```python
from build123d import *

# Parameters (mm, degrees)
SKETCH1_R                = 2.5
BOSS_EXTRUDE3_DEPTH      = 6.5
BOSS_EXTRUDE3_2_DEPTH    = 6.5
BOSS_EXTRUDE7_START      = -6.5
BOSS_EXTRUDE7_DEPTH      = 1.5
BOSS_EXTRUDE8_DEPTH      = 8.5
BOSS_EXTRUDE8_DEPTH_BACK = 8.5
SKETCH2_R                = 2.5
SKETCH3_R                = 1.5
CUT_EXTRUDE1_DEPTH       = 0.5
CUT_EXTRUDE2_START       = -0.5
SKETCH4_R                = 1.5
CUT_EXTRUDE2_DEPTH       = 0.5


with BuildPart() as part:
    # Sketch1 → Boss-Extrude3 (new, symmetric)
    with BuildSketch(Plane.XY):
        with Locations(Location((6.35, 0, 0), (0, 0, 180))):
            Circle(SKETCH1_R)
    extrude(amount=BOSS_EXTRUDE3_DEPTH, both=True)



with BuildPart() as body_2:
    # Sketch1 → Boss-Extrude3 2 (new, symmetric)
    with BuildSketch(Plane.XY):
        with Locations(Location((-6.35, 0, 0), (0, 0, 180))):
            Circle(SKETCH1_R)
    extrude(amount=BOSS_EXTRUDE3_2_DEPTH, both=True)


with BuildPart() as part_1:
    add(part.part)

    add(body_2.part)  # Boss-Extrude7 merges body 2
    # Sketch1<5> → Boss-Extrude7 (add)
    with BuildSketch(Plane.XY.offset(BOSS_EXTRUDE7_START)):
        with BuildLine():
            ThreePointArc((-3.267678659, 4.854049356), (-12.1, 0), (-3.267678659, -4.854049356))
            ThreePointArc((-3.267678659, -4.854049356), (0, -3.904220161), (3.267678659, -4.854049356))
            ThreePointArc((3.267678659, -4.854049356), (12.1, 0), (3.267678659, 4.854049356))
            ThreePointArc((3.267678659, 4.854049356), (0, 3.904220161), (-3.267678659, 4.854049356))
        make_face()
    boss_extrude7 = extrude(amount=-BOSS_EXTRUDE7_DEPTH)

    # Mirror1: Boss-Extrude7 across plane
    add(boss_extrude7.mirror(Plane.XY))

    # Sketch2 → Boss-Extrude8 (add, two sides: drawn at the far end of the back side and taken through both)
    with BuildSketch(Plane.XY.offset(-BOSS_EXTRUDE8_DEPTH_BACK)):
        with Locations(Location((-6.35, 0, 0), (0, 0, 180))):
            Circle(SKETCH2_R)
        with Locations(Location((6.35, 0, 0), (0, 0, 180))):
            Circle(SKETCH2_R)
    extrude(amount=BOSS_EXTRUDE8_DEPTH + BOSS_EXTRUDE8_DEPTH_BACK)

    # Sketch3 → Cut-Extrude1 (cut)
    with BuildSketch(Plane.XY.offset(8.5)):
        with Locations((-6.35, 0)):
            Circle(SKETCH3_R)
        with Locations((6.35, 0)):
            Circle(SKETCH3_R)
    extrude(amount=-CUT_EXTRUDE1_DEPTH, mode=Mode.SUBTRACT)

    # Sketch4 → Cut-Extrude2 (cut)
    with BuildSketch(Plane(origin=(0, 0, -8.5), x_dir=(-1, 0, 0), z_dir=(0, 0, -1)).offset(CUT_EXTRUDE2_START)):
        with Locations(Location((6.35, 0, 0), (0, 0, 180))):
            Circle(SKETCH4_R)
        with Locations(Location((-6.35, 0, 0), (0, 0, 180))):
            Circle(SKETCH4_R)
    extrude(amount=CUT_EXTRUDE2_DEPTH, mode=Mode.SUBTRACT)


solid = part_1.part
```
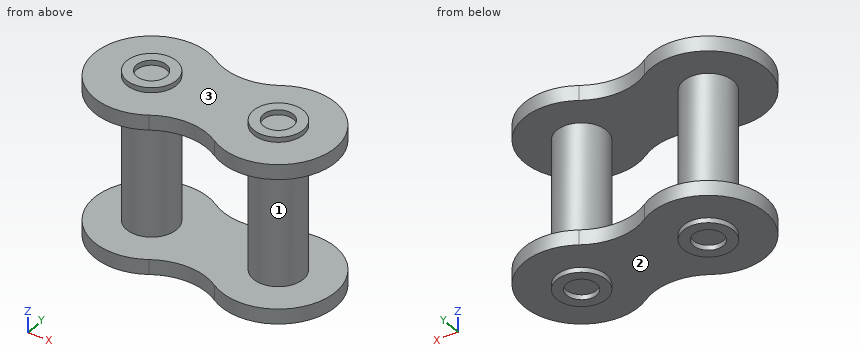
Work out the finished part from the listing and answer in its coordinate system (mm). Face numbers are marked on the shaded views. Give positions to 0.01 mm unless a question says otherwise; leave off trailing zeros. Order: outer loops, then holes, each group sorted by start corner. A loop starts at its lowest first (then second) coordinate and runs counter-clockwise, first axis right, second up. Notation, with made-up numbers: (-2, 6) - (16, 6) arc R11 ccw to (16, 11) - close; hole circle Ø9 at (56, -16.75). An arc over 180 degrees is marked (long way). One line per item, written item: value. Start each with the question number.
1. Section C-C, the plane z = -5 is taken. Write down the section's boundary in (x, y), then the cut area to 3 significant figures.
2. Consider line 1 (Y direction, x = 6.35, z = 8.3); line 2 (Z direction, x = 1.5, y = 4); line 3 (X direction, y = 2, z = -6.25). Determine where each line is inside the solid, lowest interval first.
3. Section D-D, the plane x = -6.35 is taken. Write down the section's boundary in (y, z).
4. Section A-A, the plane x = 9.5 is taken. Write down the section's boundary in (y, z).
5. Each of these flat-tipped pins is pushed along its axis until it touches: pin 1 Ø0.9 at (x, y) = (7, -0.5) entering from -Z; pin 2 Ø6 at (y, z) = (-3.5, -4.5) entering from +X; pin 3 Ø5 at (x, y) = (1, -2.5) entering from +Z. Where does it stop, or does it pass through?
6. For a pull along Z with two mould halves and no side action, classify the marked faces 1, 2 and 3 as released by +Z, released by -Z, zero draft, split by the parting line, or undercut.
Filled sheet:
1. outline: circle Ø5 at (-6.35, 0); circle Ø5 at (6.35, 0)
1. area: 39.3 mm²
2. line 1: -2.5 to -1.5, 1.5 to 2.5
2. line 2: -8 to -6.5, 6.5 to 8
2. line 3: -7.85 to -4.85, 4.85 to 7.85
3. outline: (-5.75, -8) - (-2.5, -8) - (-2.5, -8.5) - (-1.5, -8.5) - (-1.5, -8) - (1.5, -8) - (1.5, -8.5) - (2.5, -8.5) - (2.5, -8) - (5.75, -8) - (5.75, -6.5) - (2.5, -6.5) - (2.5, 6.5) - (5.75, 6.5) - (5.75, 8) - (2.5, 8) - (2.5, 8.5) - (1.5, 8.5) - (1.5, 8) - (-1.5, 8) - (-1.5, 8.5) - (-2.5, 8.5) - (-2.5, 8) - (-5.75, 8) - (-5.75, 6.5) - (-2.5, 6.5) - (-2.5, -6.5) - (-5.75, -6.5) - close
4. outline: (-4.81, -8) - (4.81, -8) - (4.81, -6.5) - (-4.81, -6.5) - close; (-4.81, 6.5) - (4.81, 6.5) - (4.81, 8) - (-4.81, 8) - close
5. pin 1: z = -8
5. pin 2: x = 11.96
5. pin 3: z = 8
6. face 1: undercut
6. face 2: released by -Z
6. face 3: released by +Z
